Source: three-view drawing plus pictorial views. Frame: mm from the lowest corner of the part. Give positions to 0.01 mm unless a question says otherwise; leave off trailing zeros. Order: outer loops, then holes, each group sorted by start corner. A loop starts at its lowest first (then second) coordinate and runs counter-clockwise, first axis right, second up. Notation, with made-up numbers: (62.5, -9) -> (86.5, -9) arc R35 ccw to (86.5, 23) -> close; hole circle Ø11 at (71.25, 31.5). An arc over 180 degrees is marked (long way). Answer in a Markdown table with one row per item.
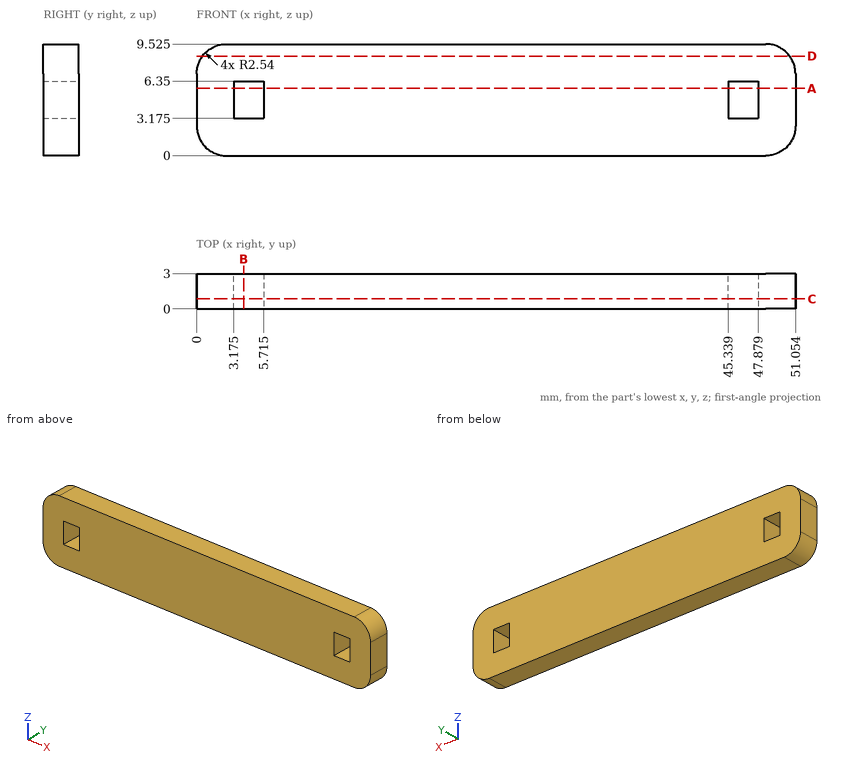
(1) Section query B-B (x = 4). Return the cut outline in (y, z) (3 decimals).
A:
| item | result |
|---|---|
| outline | (0, 0) -> (3, 0) -> (3, 3.175) -> (0, 3.175) -> close; (0, 6.35) -> (3, 6.35) -> (3, 9.525) -> (0, 9.525) -> close |
(2) Section query A-A (z = 5.75). Return the cut outline in (x, y) (3 decimals), plus the area to 3 significant figures.
A:
| item | result |
|---|---|
| outline | (0, 0) -> (3.175, 0) -> (3.175, 3) -> (0, 3) -> close; (5.715, 0) -> (45.339, 0) -> (45.339, 3) -> (5.715, 3) -> close; (47.879, 0) -> (51.054, 0) -> (51.054, 3) -> (47.879, 3) -> close |
| area | 138 mm^2 |
(3) Ray query, probe 1 along X at (y, z) = (0.6, 5.25) (3 decimals); probe 2 along X at (y, z) = (1.15, 8.25); probe 3 along X at (y, z) = (0.8, 1.75). Return the intervals inside material, ascending.
A:
| item | result |
|---|---|
| probe 1 | x = 0 to 3.175, 5.715 to 45.339, 47.879 to 51.054 |
| probe 2 | x = 0.34 to 50.72 |
| probe 3 | x = 0.13 to 50.93 |
(4) Section query D-D (z = 8.5). Return the cut outline in (x, y).
A:
| item | result |
|---|---|
| outline | (0.5, 0) -> (50.55, 0) -> (50.55, 3) -> (0.5, 3) -> close |
(5) Section query C-C (y = 0.85). Return the cut outline in (x, z) (3 decimals).
A:
| item | result |
|---|---|
| outline | (0, 2.54) arc R2.54 ccw to (2.54, 0) -> (48.514, 0) arc R2.54 ccw to (51.054, 2.54) -> (51.054, 6.985) arc R2.54 ccw to (48.514, 9.525) -> (2.54, 9.525) arc R2.54 ccw to (0, 6.985) -> close; hole (3.175, 3.175) -> (5.715, 3.175) -> (5.715, 6.35) -> (3.175, 6.35) -> close; hole (45.339, 3.175) -> (47.879, 3.175) -> (47.879, 6.35) -> (45.339, 6.35) -> close |
